Could you check a few things on this drawing? It's one solid part, dimensions in mm from its lowest x, y, z. Give positions to 0.01 mm unless a question says otherwise; leave off trailing zeros. Order: outer loops, then holes, each group sorted by start corner. A loop starts at its lowest first (then second) coordinate and runs counter-clockwise, first axis right, second up. Notation, with made-up numbers: (12, 79.5) - (18, 79.5) arc R10 cw to (18, 87.5) - close; hole circle Ø5 at (38.25, -25.5). An arc over 180 degrees is marked (long way). Return JSON: item names as keys, results as strings.
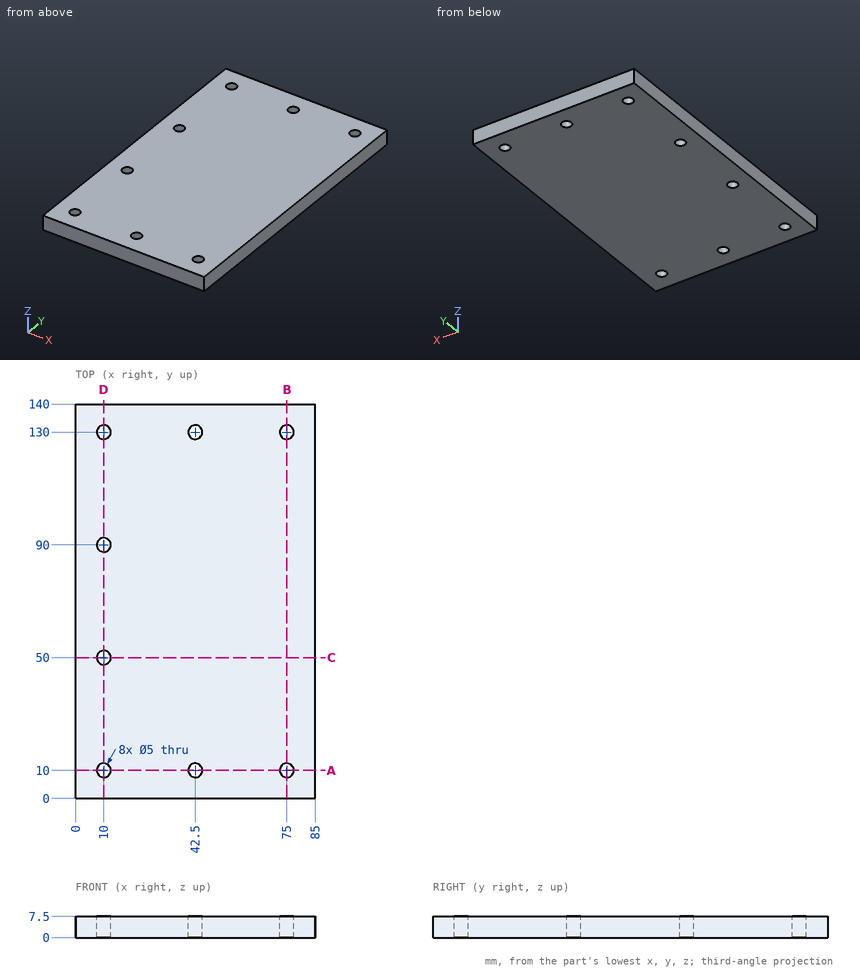
1. Suppose I cut it at C-C (y = 50). List the corners of the cut face in (x, z) for me, plus the area to 3 significant figures.
Checks:
{"outline": "(0, 0) - (7.5, 0) - (7.5, 7.5) - (0, 7.5) - close; (12.5, 0) - (85, 0) - (85, 7.5) - (12.5, 7.5) - close", "area": "600 mm^2"}
2. If I drill on L1, parallel to Y at x = 75, z = 5; L2, parallel to Y at x = 10, z = 3.5; L3, parallel to X at y = 130, z = 5.5, over which ranges is the centre line in solid material (lowest first)? Write a range as [from, to].
Checks:
{"L1": "[0, 7.5], [12.5, 127.5], [132.5, 140]", "L2": "[0, 7.5], [12.5, 47.5], [52.5, 87.5], [92.5, 127.5], [132.5, 140]", "L3": "[0, 7.5], [12.5, 40], [45, 72.5], [77.5, 85]"}
3. Suppose I cut it at A-A (y = 10). List the corners of the cut face in (x, z) for me.
Checks:
{"outline": "(0, 0) - (7.5, 0) - (7.5, 7.5) - (0, 7.5) - close; (12.5, 0) - (40, 0) - (40, 7.5) - (12.5, 7.5) - close; (45, 0) - (72.5, 0) - (72.5, 7.5) - (45, 7.5) - close; (77.5, 0) - (85, 0) - (85, 7.5) - (77.5, 7.5) - close"}
4. Suppose I cut it at D-D (x = 10). List the corners of the cut face in (y, z) for me.
Checks:
{"outline": "(0, 0) - (7.5, 0) - (7.5, 7.5) - (0, 7.5) - close; (12.5, 0) - (47.5, 0) - (47.5, 7.5) - (12.5, 7.5) - close; (52.5, 0) - (87.5, 0) - (87.5, 7.5) - (52.5, 7.5) - close; (92.5, 0) - (127.5, 0) - (127.5, 7.5) - (92.5, 7.5) - close; (132.5, 0) - (140, 0) - (140, 7.5) - (132.5, 7.5) - close"}
5. Suppose I cut it at B-B (x = 75). List the corners of the cut face in (y, z) for me, plus the area to 3 significant figures.
Checks:
{"outline": "(0, 0) - (7.5, 0) - (7.5, 7.5) - (0, 7.5) - close; (12.5, 0) - (127.5, 0) - (127.5, 7.5) - (12.5, 7.5) - close; (132.5, 0) - (140, 0) - (140, 7.5) - (132.5, 7.5) - close", "area": "975 mm^2"}
